Check sheet for the modelled part. Datum: model origin and axes. Units: mm. Give positions to 0.01 mm unless a question says otherwise; leave off trailing zeros. Order: outer loops, then holes, each group sorted by start corner. A loop starts at its lowest first (then second) coordinate and runs counter-clockwise, first axis right, second up. Notation, with made-up numbers: M 6.5,29 L 49.5,29 A33 cw 49.5,67 Z; hole C 19,33.25 d6. An arc over 180 degrees is marked long. Answer in a Markdown table with one row per item. Add a question column.
from build123d import *

# Parameters (mm, degrees)
ESQUISSE1_W                = 100
ESQUISSE1_H                = 100
BOSS_EXTRU_1_DEPTH         = 200
ESQUISSE2_W                = 80
ESQUISSE2_H                = 180
ENL_V_MAT_EXTRU_1_DEPTH    = 15
ESQUISSE3_W                = 15
ESQUISSE3_H                = 15
BOSS_EXTRU_2_DEPTH         = 80
R_P_TITION_LIN_AIRE1_COUNT = 6
R_P_TITION_LIN_AIRE1_PITCH = 20
ESQUISSE4_W                = 50
ESQUISSE4_H                = 5
ESQUISSE4_W_2              = 7
ESQUISSE4_H_2              = 4
ENL_V_MAT_EXTRU_2_DEPTH    = 2
R_P_TITION_LIN_AIRE2_COUNT = 6
R_P_TITION_LIN_AIRE2_PITCH = 20
ESQUISSE5_W                = 25
ESQUISSE5_H                = 15
BOSS_EXTRU_3_DEPTH         = 60
ESQUISSE6_W                = 15
ESQUISSE6_H                = 15
BOSS_EXTRU_4_DEPTH         = 50
R_P_TITION_LIN_AIRE3_COUNT = 2
R_P_TITION_LIN_AIRE3_PITCH = 30
ESQUISSE7_W                = 6
ESQUISSE7_H                = 45
ESQUISSE7_W_2              = 35
ESQUISSE7_H_2              = 5
ENL_V_MAT_EXTRU_3_DEPTH    = 3


with BuildPart() as part:
    # Esquisse1 → Boss.-Extru.1 (new body)
    with BuildSketch(Plane.XY):
        Rectangle(ESQUISSE1_W, ESQUISSE1_H)
    extrude(amount=BOSS_EXTRU_1_DEPTH)

    # Esquisse2 → Enlèv. mat.-Extru.1 (cut)
    with BuildSketch(Plane.XZ.offset(50)):
        with Locations((0, 100)):
            Rectangle(ESQUISSE2_W, ESQUISSE2_H)
    extrude(amount=-ENL_V_MAT_EXTRU_1_DEPTH, mode=Mode.SUBTRACT)

    # Esquisse3 → Boss.-Extru.2 (add)
    with BuildSketch(Plane(origin=(-40, 0, 0), x_dir=(0, 0, -1), z_dir=(1, 0, 0))):
        with Locations((-177.5, -42.5)):
            Rectangle(ESQUISSE3_W, ESQUISSE3_H)
    boss_extru_2 = extrude(amount=BOSS_EXTRU_2_DEPTH)

    # Répétition linéaire1: Boss.-Extru.2 ×6
    with Locations(*[(0, 0, -i * R_P_TITION_LIN_AIRE1_PITCH) for i in range(1, R_P_TITION_LIN_AIRE1_COUNT)]):
        add(boss_extru_2)

    # Esquisse4 → Enlèv. mat.-Extru.2 (cut)
    with BuildSketch(Plane.XZ.offset(50)):
        with Locations((-15, 177.5)):
            Rectangle(ESQUISSE4_W, ESQUISSE4_H)
        with Locations((21.5, 181)):
            Rectangle(ESQUISSE4_W_2, ESQUISSE4_H_2)
        with Locations((21.5, 174)):
            Rectangle(ESQUISSE4_W_2, ESQUISSE4_H_2)
    enl_v_mat_extru_2 = extrude(amount=-ENL_V_MAT_EXTRU_2_DEPTH, mode=Mode.SUBTRACT)

    # Répétition linéaire2: Enlèv. mat.-Extru.2 ×6
    with Locations(*[(0, 0, -i * R_P_TITION_LIN_AIRE2_PITCH) for i in range(1, R_P_TITION_LIN_AIRE2_COUNT)]):
        add(enl_v_mat_extru_2, mode=Mode.SUBTRACT)

    # Esquisse5 → Boss.-Extru.3 (add)
    with BuildSketch(Plane(origin=(0, 0, 70), x_dir=(-1, 0, 0), z_dir=(0, 0, -1))):
        with Locations((22.5, -42.5)):
            Rectangle(ESQUISSE5_W, ESQUISSE5_H)
    extrude(amount=BOSS_EXTRU_3_DEPTH)

    # Esquisse6 → Boss.-Extru.4 (add)
    with BuildSketch(Plane(origin=(-10, 0, 0), x_dir=(0, 0, -1), z_dir=(1, 0, 0))):
        with Locations((-57.5, -42.5)):
            Rectangle(ESQUISSE6_W, ESQUISSE6_H)
    boss_extru_4 = extrude(amount=BOSS_EXTRU_4_DEPTH)

    # Répétition linéaire3: Boss.-Extru.4 ×2
    with Locations(*[(0, 0, -i * R_P_TITION_LIN_AIRE3_PITCH) for i in range(1, R_P_TITION_LIN_AIRE3_COUNT)]):
        add(boss_extru_4)

    # Esquisse7 → Enlèv. mat.-Extru.3 (cut)
    with BuildSketch(Plane.XZ.offset(50)):
        with Locations((-26, 32.5)):
            Rectangle(ESQUISSE7_W, ESQUISSE7_H)
        with Locations((7.5, 57.5)):
            Rectangle(ESQUISSE7_W_2, ESQUISSE7_H_2)
        with Locations((7.5, 27.5)):
            Rectangle(ESQUISSE7_W_2, ESQUISSE7_H_2)
    extrude(amount=-ENL_V_MAT_EXTRU_3_DEPTH, mode=Mode.SUBTRACT)


solid = part.part
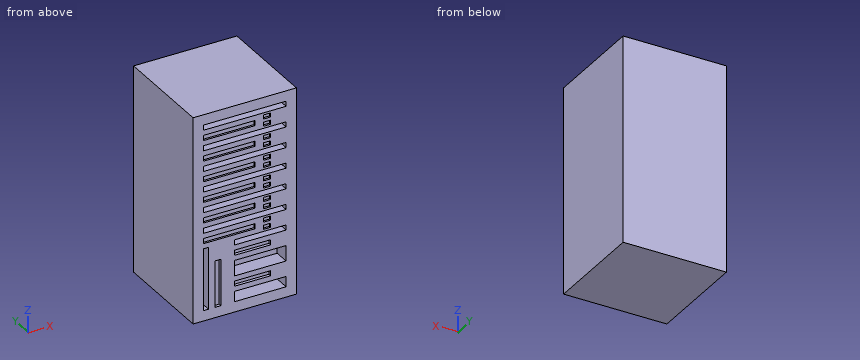
Q1. Go/stop test with flat-tipped pins: pin 1 (2.5 mm diameter, centred on x = -8, z = 148.5, fed in from -Y); pin 2 (2 mm diameter, centred on x = 20, z = 114.5, fed in from -Y). Record where each tip stops, or that it passes through.
Q2. Cross-section at B-B (y = -41). State how many separate pieces and enclosed holes the cut face has, and give its area (3 significant figures).
Q3. Thickness scan on probe 1 along X at (y, z) = (-44.5, 36); probe 2 along Y at (x, z) = (24.5, 153); probe 3 along Y at (x, z) = (-26, 12.5). Record the ranges inside material, lowest first.
Q4. Cross-section at A-A (z = 18). Record the boundary of the cut face in (x, y), and give its area (3 significant figures).
Values follow:
| question | item | result |
|---|---|---|
| 1 | pin 1 | y = -35 |
| 1 | pin 2 | y = -48 |
| 2 | separate pieces | 1 |
| 2 | enclosed holes | 10 |
| 2 | area | 15,800 mm² |
| 3 | probe 1 | -50 to -40, -35 to -10, 40 to 50 |
| 3 | probe 2 | -48 to 50 |
| 3 | probe 3 | -47 to 50 |
| 4 | outline | M -50,-50 L -40,-50 L -40,-35 L -35,-35 L -35,-50 L -29,-50 L -29,-47 L -23,-47 L -23,-50 L -10,-50 L -10,-35 L 40,-35 L 40,-50 L 50,-50 L 50,50 L -50,50 Z |
| 4 | area | 9,160 mm² |
